Check sheet for the modelled part. Datum: model origin and axes. Units: mm. A direction names the side the tool comes from. Give positions to 0.01 mm unless a question says otherwise; leave off trailing zeros. Loops run counter-clockwise (first coordinate to the right, second up) from the corner with the lowest first, then second, coordinate; pieces in that order, holes last.
```python
from build123d import *

# Parameters (mm, degrees)
F0_R     = 1.27
F0_R_2   = 1.7145
F1_DEPTH = 2.54
F3_DEPTH = 1.524
F4_R     = 1
F6_DEPTH = 1.27
F7_W     = 10
F7_H     = 10
F8_DEPTH = 4.572
F9_R     = 5


with BuildPart() as f1:
    # F0 (on Top) → F1 (new body)
    with BuildSketch(Plane.XY):
        with BuildLine():
            Line((39.37, 33.6385), (-39.37, 33.6385))
            ThreePointArc((-39.37, 33.6385), (-42.905534, 32.174034), (-44.37, 28.6385))
            Line((-44.37, 28.6385), (-44.37, -28.6385))
            ThreePointArc((-44.37, -28.6385), (-42.905534, -32.174034), (-39.37, -33.6385))
            Line((-39.37, -33.6385), (39.37, -33.6385))
            ThreePointArc((39.37, -33.6385), (42.905534, -32.174034), (44.37, -28.6385))
            Line((44.37, -28.6385), (44.37, 28.6385))
            ThreePointArc((44.37, 28.6385), (42.905534, 32.174034), (39.37, 33.6385))
        make_face()
        with Locations((-19.779271, -13.6525)):
            Circle(F0_R, mode=Mode.SUBTRACT)
        Polygon((39.079527, -24.384), (37.319764, -27.432), (33.800236, -27.432), (32.040473, -24.384), (33.800236, -21.336), (37.319764, -21.336), align=None, mode=Mode.SUBTRACT)
        with Locations((11.589729, -13.6525)):
            Circle(F0_R, mode=Mode.SUBTRACT)
        with Locations((-19.779271, 13.6525)):
            Circle(F0_R, mode=Mode.SUBTRACT)
        with Locations((11.589729, 13.6525)):
            Circle(F0_R, mode=Mode.SUBTRACT)
        Polygon((39.079527, 24.384), (37.319764, 21.336), (33.800236, 21.336), (32.040473, 24.384), (33.800236, 27.432), (37.319764, 27.432), align=None, mode=Mode.SUBTRACT)
        Polygon((33.800236, 21.336), (37.319764, 21.336), (39.079527, 24.384), (37.319764, 27.432), (33.800236, 27.432), (32.040473, 24.384), align=None)
        with Locations((35.56, 24.384)):
            Circle(F0_R_2, mode=Mode.SUBTRACT)
        Polygon((33.800236, -27.432), (37.319764, -27.432), (39.079527, -24.384), (37.319764, -21.336), (33.800236, -21.336), (32.040473, -24.384), align=None)
        with Locations((35.56, -24.384)):
            Circle(F0_R_2, mode=Mode.SUBTRACT)
    extrude(amount=F1_DEPTH)

    # F2 (on face) → F3 (cut)
    with BuildSketch(Plane(origin=(0, 0, 0), x_dir=(1, 0, 0), z_dir=(0, 0, -1))):
        with BuildLine():
            Line((11.399229, 16.764), (-19.588771, 16.764))
            ThreePointArc((-19.588771, 16.764), (-21.923637, 15.796867), (-22.890771, 13.462))
            Line((-22.890771, 13.462), (-22.890771, -13.462))
            ThreePointArc((-22.890771, -13.462), (-21.923637, -15.796867), (-19.588771, -16.764))
            Line((-19.588771, -16.764), (11.399229, -16.764))
            ThreePointArc((11.399229, -16.764), (13.734096, -15.796867), (14.701229, -13.462))
            Line((14.701229, -13.462), (14.701229, 13.462))
            ThreePointArc((14.701229, 13.462), (13.734096, 15.796867), (11.399229, 16.764))
        make_face()
        with BuildLine():
            Line((-21.239771, -10.471786), (-21.239771, 10.471786))
            ThreePointArc((-21.239771, 10.471786), (-17.304397, 11.177626), (-16.598557, 15.113))
            Line((-16.598557, 15.113), (8.409016, 15.113))
            ThreePointArc((8.409016, 15.113), (9.114856, 11.177626), (13.050229, 10.471786))
            Line((13.050229, 10.471786), (13.050229, -10.471786))
            ThreePointArc((13.050229, -10.471786), (9.114856, -11.177626), (8.409016, -15.113))
            Line((8.409016, -15.113), (-16.598557, -15.113))
            ThreePointArc((-16.598557, -15.113), (-17.304397, -11.177626), (-21.239771, -10.471786))
        make_face(mode=Mode.SUBTRACT)
    extrude(amount=-F3_DEPTH, mode=Mode.SUBTRACT)

    # F4
    f4_edges = [f1.edges().sort_by_distance(p)[0] for p in [
        (-17.304397, 11.177626, 0),
        (-4.094771, 15.113, 0),
        (9.114856, 11.177626, 0),
        (13.050229, 0, 0),
        (9.114856, -11.177626, 0),
        (-4.094771, -15.113, 0),
        (-17.304397, -11.177626, 0),
        (-21.239771, 0, 0),
        (-22.890771, 0, 0),
        (-21.923637, -15.796867, 0),
    ]]
    fillet(f4_edges, radius=F4_R)

    # F5 (on face) → F6 (cut)
    with BuildSketch(Plane.XY.offset(2.54)):
        Polygon((33.800236, 27.432), (32.040473, 24.384), (33.800236, 21.336), (37.319764, 21.336), (39.079527, 24.384), (37.319764, 27.432), align=None)
        Polygon((33.800236, -21.336), (32.040473, -24.384), (33.800236, -27.432), (37.319764, -27.432), (39.079527, -24.384), (37.319764, -21.336), align=None)
    extrude(amount=-F6_DEPTH, mode=Mode.SUBTRACT)

    # F7 (on face) → F8 (join)
    with BuildSketch(Plane.XY.offset(2.54)):
        with Locations((-27.051, 19.05)):
            Rectangle(F7_W, F7_H)
        with Locations((-27.051, -19.05)):
            Rectangle(F7_W, F7_H)
    extrude(amount=F8_DEPTH)

    # F9
    f9_edges = [f1.edges().sort_by_distance(p)[0] for p in [
        (-22.051, -14.05, 4.826),
        (-22.051, 14.05, 4.826),
    ]]
    fillet(f9_edges, radius=F9_R)


solid = f1.part
```
(1) Section check A-A on x = 35.56. Record the boundary of the cut face in (y, z).
(2) Section check B-B on z = 4. Record the boundary of the cut face in (x, y).
(3) Material ranges on line 1 (X direction, y = 5.5, z = 1.25); line 2 (Y direction, x = -28, z = 2.75); line 3 (Z direction, x = 24.5, y = -16.5), recorded low to high.
(4) Access from +Z, -Z, +X, -X, +Y, -Y to the whole of each face (thin tool, end or side, straight path). Record for faces 4 (the face through (13.71, 15.82, 1.26)), 5 (the face through (38.187, -25.929, 1.914)), 6 (the face through (-30, 14.05, 5)).
(5) Gauge pin test, flat ends, axial feed: pin 1 Ø3 at (x, y) = (11.59, 13.65) entering from -Z; pin 2 Ø3.5 at (y, z) = (-18.5, 5.5) entering from -X; pin 3 Ø4 at (x, y) = (24, 8.5) entering from +Z. Record the tip position at first contact, or that the pin passes through.
(6) Section check C-C on y = -5.5. Record the boundary of the cut face in (x, z), plus the area to 3 significant figures.
(7) Release check for a two-part mould opening along Y. For faces 1 (the face through (32.91, -25.89, 1.91)), 2 (the face through (-32.051, -19, 5)), 3 (the face through (-42.87, 32.21, 1.25)) record: pulls with the +Y half, pulls with the -Y half, needs draft (parallel to the pull), parting line crosses it, or undercut.
Computed values:
1. outline: (-33.64, 0) - (-26.1, 0) - (-26.1, 1.27) - (-27.43, 1.27) - (-27.43, 2.54) - (-33.64, 2.54) - close; (-22.67, 0) - (22.67, 0) - (22.67, 1.27) - (21.34, 1.27) - (21.34, 2.54) - (-21.34, 2.54) - (-21.34, 1.27) - (-22.67, 1.27) - close; (26.1, 0) - (33.64, 0) - (33.64, 2.54) - (27.43, 2.54) - (27.43, 1.27) - (26.1, 1.27) - close
2. outline: (-32.05, -24.05) - (-22.05, -24.05) - (-22.05, -19.05) arc R5 ccw to (-27.05, -14.05) - (-32.05, -14.05) - close; (-32.05, 14.05) - (-27.05, 14.05) arc R5 ccw to (-22.05, 19.05) - (-22.05, 24.05) - (-32.05, 24.05) - close
3. line 1: x = -44.37 to -22.89, -21.24 to 13.05, 14.7 to 44.37
3. line 2: y = -24.05 to -14.05, 14.05 to 24.05
3. line 3: z = 0 to 2.54
4. face 4: -Z
4. face 5: +Z
4. face 6: +Z, +X, -X
5. pin 1: stops at z = 1.52
5. pin 2: stops at x = -32.05
5. pin 3: stops at z = 2.54
6. outline: (-44.37, 0) - (-23.89, 0) arc R1 ccw to (-22.89, 1) - (-22.89, 1.52) - (-21.24, 1.52) - (-21.24, 1) arc R1 ccw to (-20.24, 0) - (12.05, 0) arc R1 ccw to (13.05, 1) - (13.05, 1.52) - (14.7, 1.52) - (14.7, 1) arc R1 ccw to (15.7, 0) - (44.37, 0) - (44.37, 2.54) - (-44.37, 2.54) - close
6. area: 220 mm2
7. face 1: undercut
7. face 2: needs draft
7. face 3: pulls with the +Y half
